Design review of the part shown in the three views and the two pictorial views. Dimensions are in mm from the part's minimum x, y and z. A direction names the side the tool comes from. Coordinates: 2 decimals unless noted, no trailing zeros. Write each loop counter-clockwise with the first axis right and the second up, starting at its lowest first coordinate (ties: lowest second). Pieces come first, ordered by that corner, then holes. Notation, with made-up numbers: (48, 72) -> (61, 72) arc R11 ccw to (61, 88) -> close; hole circle Ø6 at (74, 71.25). An arc over 180 degrees is marked (long way). Write each question's results on one line, items separated by ' | '.
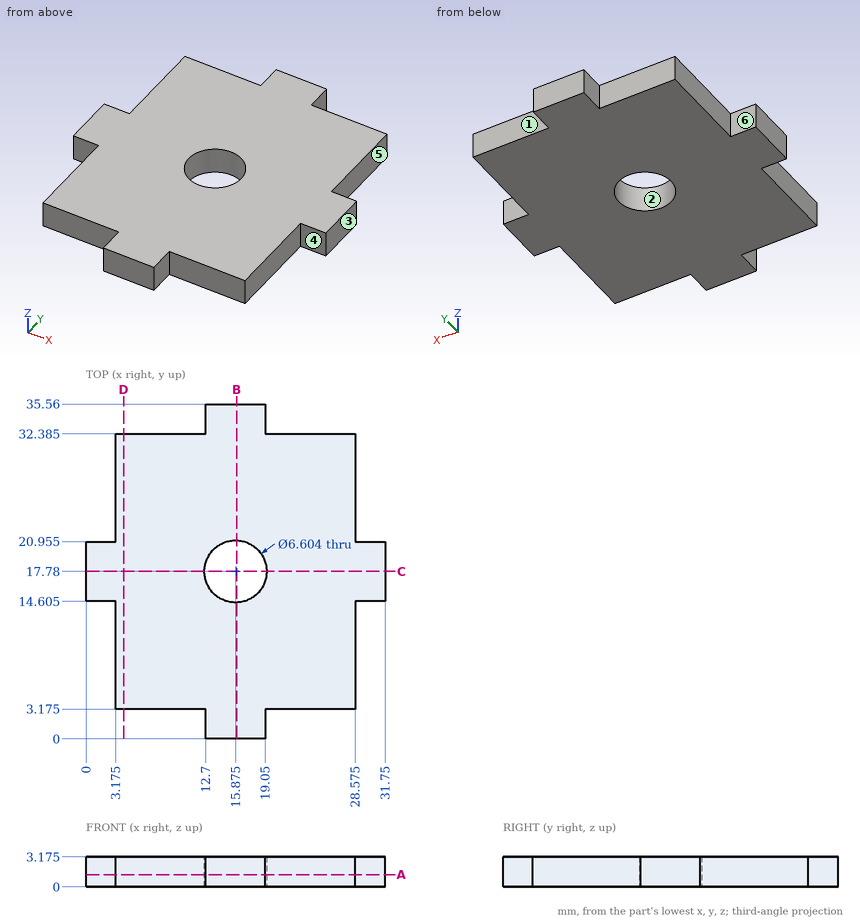
Q1. Add section A-A (z = 1.3). Write out the cut boundary in (x, y) (3 decimals), plus the area to 3 significant figures.
Solution:
outline: (0, 14.605) -> (3.175, 14.605) -> (3.175, 3.175) -> (12.7, 3.175) -> (12.7, 0) -> (19.05, 0) -> (19.05, 3.175) -> (28.575, 3.175) -> (28.575, 14.605) -> (31.75, 14.605) -> (31.75, 20.955) -> (28.575, 20.955) -> (28.575, 32.385) -> (19.05, 32.385) -> (19.05, 35.56) -> (12.7, 35.56) -> (12.7, 32.385) -> (3.175, 32.385) -> (3.175, 20.955) -> (0, 20.955) -> close; hole circle Ø6.604 at (15.875, 17.78) | area: 788 mm²
Q2. Add section B-B (x = 16). Write out the cut boundary in (y, z) (3 decimals), plus the area to 3 significant figures.
Solution:
outline: (0, 0) -> (14.48, 0) -> (14.48, 3.175) -> (0, 3.175) -> close; (21.08, 0) -> (35.56, 0) -> (35.56, 3.175) -> (21.08, 3.175) -> close | area: 92.0 mm²
Q3. Draft analysis for pull direction X (two halves, no side actions). For the marked faces 1, 2 and 3, state which applies: pulls with the +X half, pulls with the -X half, needs draft (parallel to the pull), parting line crosses it, or undercut.
Solution:
face 1: needs draft | face 2: undercut | face 3: pulls with the +X half
Q4. Add section D-D (x = 4). Write out the cut boundary in (y, z) (3 decimals).
Solution:
outline: (3.175, 0) -> (32.385, 0) -> (32.385, 3.175) -> (3.175, 3.175) -> close
Q5. For line 1 (Y direction, x = 16, z = 0.85); line 2 (Y direction, x = 5, z = 0.25) (3 decimals); line 3 (Y direction, x = 13, z = 0.3), list the stretches that pass through material, from the lowest coordinate up. Write a range as from..to.
Solution:
line 1: 0..14.48, 21.08..35.56 | line 2: 3.175..32.385 | line 3: 0..16.16, 19.4..35.56
Q6. Machinability: for the marked faces 4, 5 and 6, which of the approach directions +Z, -Z, +X, -X, +Y, -Y give a long, thin tool a straight path to every point of the face, cutting with its end or side? Answer none if there is none.
Solution:
face 4: +Z, -Z, +X, -Y | face 5: +Z, -Z, +X, +Y | face 6: +Z, -Z, -X, +Y
Q7. Add section C-C (y = 17.78). Write out the cut boundary in (x, z) (3 decimals).
Solution:
outline: (0, 0) -> (12.573, 0) -> (12.573, 3.175) -> (0, 3.175) -> close; (19.177, 0) -> (31.75, 0) -> (31.75, 3.175) -> (19.177, 3.175) -> close
Q8. Clearance check with flat-ended pins moving along their axes: P1, Ø1.6, axis at x = 30.5, z = 1, coming from the +Y side (3 decimals); P2, Ø1.5, axis at x = 27, z = 2.5, coming from the -Y side (3 decimals). State where each tip first meets the part, or that it passes through.
Solution:
P1: y = 20.955 | P2: y = 3.175
